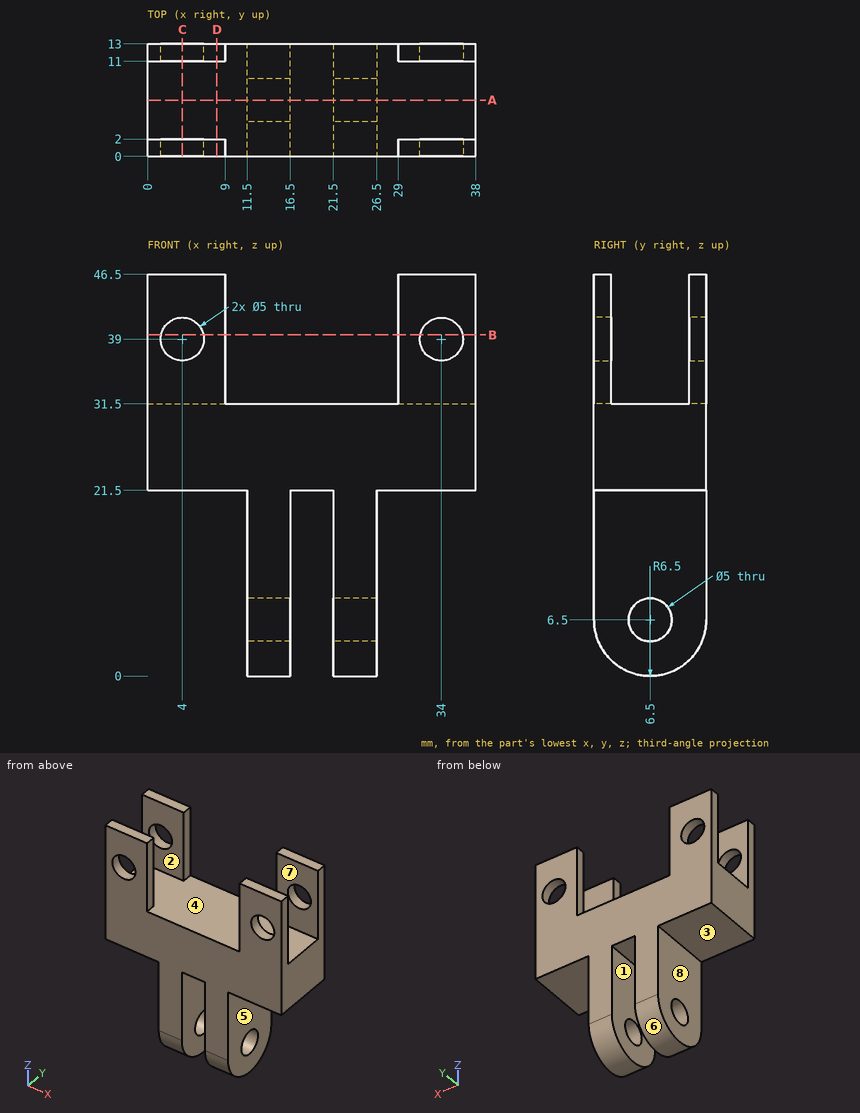
Can you work these out from the drawing? Everything is in mm from the part's minimum corner. A direction names the side the tool comes from. Round coordinates to 2 decimals unless told otherwise and drop trailing zeros. Loops run counter-clockwise (first coordinate to the right, second up) from the corner with the lowest first, then second, coordinate; pieces in that order, holes last. Notation, with made-up numbers: (22.5, 55) -> (26.5, 55) arc R28 ccw to (26.5, 89) -> close; hole circle Ø3 at (84.5, 75.5). An arc over 180 degrees is marked (long way). Put each result on its own line as item: value.
Q1. I want a section at B-B on z = 39.5. Give the number of separate pieces and of enclosed holes in the cut face, and give its area (3 significant figures).
Checks:
separate pieces: 8
enclosed holes: 0
area: 32.8 mm2
Q2. I want a section at D-D on x = 8. Write out the boundary of the cut face in (y, z).
Checks:
outline: (0, 21.5) -> (13, 21.5) -> (13, 46.5) -> (11, 46.5) -> (11, 31.5) -> (2, 31.5) -> (2, 46.5) -> (0, 46.5) -> close
Q3. Please list where these lines run through material, in increasing order: line 1 (X direction, y = 11.8, z = 39); line 2 (Y direction, x = 23.7, z = 6.5); line 3 (Z direction, x = 34, y = 1.1). Write a range as from..to.
Checks:
line 1: 0..1.5, 6.5..9, 29..31.5, 36.5..38
line 2: 0..4, 9..13
line 3: 21.5..36.5, 41.5..46.5
Q4. For pin 1 Ø6 at (x, y) = (6, 4.5) entering from -Z; pin 2 Ø3 at (x, y) = (33.5, 7) entering from +Z; pin 3 Ø6.5 at (y, z) = (6.5, 6.5) entering from -X, each with a flat end and sliding along its axis, tell me the tip position at first contact or that it passes through.
Checks:
pin 1: z = 21.5
pin 2: z = 31.5
pin 3: x = 11.5
Q5. Which directions (+Z, -Z, +X, -X, +Y, -Y) give clear straight access to the entire face, cutting with the end or side of a thin tool? Please do the marked faces 1, 2, 3, 4 and 5.
Checks:
face 1: -Z, +Y, -Y
face 2: +Z, +X, -X
face 3: -Z, -X, +Y, -Y
face 4: +Z
face 5: -Z, +X, +Y, -Y
Q6. I want a section at A-A on y = 6.5. Write out the boundary of the cut face in (x, z).
Checks:
outline: (0, 21.5) -> (11.5, 21.5) -> (11.5, 9) -> (16.5, 9) -> (16.5, 21.5) -> (21.5, 21.5) -> (21.5, 9) -> (26.5, 9) -> (26.5, 21.5) -> (38, 21.5) -> (38, 31.5) -> (0, 31.5) -> close; (11.5, 0) -> (16.5, 0) -> (16.5, 4) -> (11.5, 4) -> close; (21.5, 0) -> (26.5, 0) -> (26.5, 4) -> (21.5, 4) -> close
Q7. I want a section at C-C on x = 4. Write out the boundary of the cut face in (y, z), and give its area (3 significant figures).
Checks:
outline: (0, 21.5) -> (13, 21.5) -> (13, 36.5) -> (11, 36.5) -> (11, 31.5) -> (2, 31.5) -> (2, 36.5) -> (0, 36.5) -> close; (0, 41.5) -> (2, 41.5) -> (2, 46.5) -> (0, 46.5) -> close; (11, 41.5) -> (13, 41.5) -> (13, 46.5) -> (11, 46.5) -> close
area: 170 mm2
Q8. Thinking about a two-plate mould opening in Y: for the marked faces 6, 7 and 8, which applies, pulls with the +Y half, pulls with the -Y half, needs draft (parallel to the pull), parting line crosses it, or undercut?
Checks:
face 6: parting line crosses it
face 7: undercut
face 8: needs draft
